For this review, take the finished solid that the model builds, in its own axes (mm). Face numbers are marked on the shaded views. A direction names the side the tool comes from. Coordinates: 2 decimals unless noted, no trailing zeros. Order: outer loops, then holes, each group sorted by start corner. A loop starts at its lowest first (then second) coordinate and runs counter-clockwise, first axis right, second up.
from build123d import *

# Parameters (mm, degrees)
CROQUIS1_R                     = 12.5
CROQUIS1_R_2                   = 11
SALIENTE_EXTRUIR1_DEPTH        = 4
SALIENTE_EXTRUIR1_DEPTH_BACK   = 4
CROQUIS1_R_3                   = 6.5
CROQUIS1_R_4                   = 5
SALIENTE_EXTRUIR1_2_DEPTH      = 4
SALIENTE_EXTRUIR1_2_DEPTH_BACK = 4
CROQUIS1_4_R                   = 11
CROQUIS1_4_R_2                 = 6.5
SALIENTE_EXTRUIR2_DEPTH        = 3.5
SALIENTE_EXTRUIR2_DEPTH_BACK   = 3.5


with BuildPart() as part:
    # Croquis1 → Saliente-Extruir1 (new body, two sides)
    with BuildSketch(Plane.XY) as saliente_extruir1_sk:
        Circle(CROQUIS1_R)
        Circle(CROQUIS1_R_2, mode=Mode.SUBTRACT)
    extrude(amount=SALIENTE_EXTRUIR1_DEPTH)
    extrude(saliente_extruir1_sk.sketch, amount=-SALIENTE_EXTRUIR1_DEPTH_BACK)



with BuildPart() as body_2:
    # Croquis1 → Saliente-Extruir1 2 (new body, two sides)
    with BuildSketch(Plane.XY) as saliente_extruir1_2_sk:
        Circle(CROQUIS1_R_3)
        Circle(CROQUIS1_R_4, mode=Mode.SUBTRACT)
    extrude(amount=SALIENTE_EXTRUIR1_2_DEPTH)
    extrude(saliente_extruir1_2_sk.sketch, amount=-SALIENTE_EXTRUIR1_2_DEPTH_BACK)


with BuildPart() as part_1:
    add(part.part)

    add(body_2.part)  # Saliente-Extruir2 merges body 2
    # Croquis1_4 → Saliente-Extruir2 (add, two sides)
    with BuildSketch(Plane.XY) as saliente_extruir2_sk:
        Circle(CROQUIS1_4_R)
        Circle(CROQUIS1_4_R_2, mode=Mode.SUBTRACT)
    extrude(amount=SALIENTE_EXTRUIR2_DEPTH)
    extrude(saliente_extruir2_sk.sketch, amount=-SALIENTE_EXTRUIR2_DEPTH_BACK)


solid = part_1.part
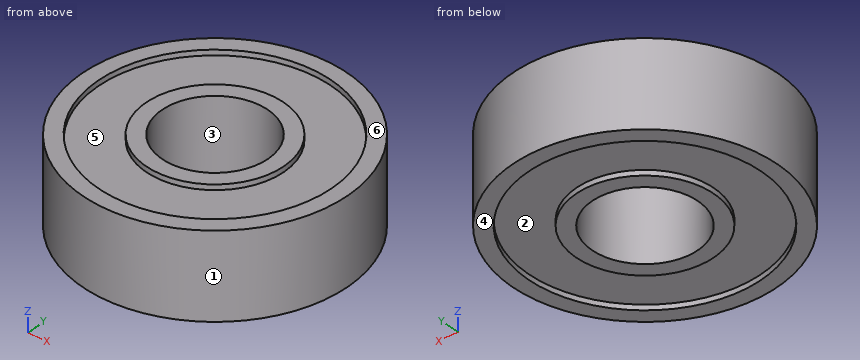
1. Clearance check with flat-ended pins moving along their axes: pin 1 Ø1.5 at (x, y) = (-9, -5.5) entering from +Z; pin 2 Ø2 at (x, y) = (-8, 5.5) entering from -Z; pin 3 Ø6 at (x, y) = (0, 0) entering from -Z. State where each tip first meets the part, or that it passes through.
Answer below:
pin 1: stops at z = 4
pin 2: stops at z = -3.5
pin 3: passes through
2. Take a section at D-D, the plane z = 0.25. Give the boundary of the cut face in (x, y).
Answer below:
outline: circle Ø25 at (0, 0); hole circle Ø10 at (0, 0)
3. Machinability: for the marked faces 5 and 6, which of the approach directions +Z, -Z, +X, -X, +Y, -Y give a long, thin tool a straight path to every point of the face, cutting with its end or side? Answer none if there is none.
Answer below:
face 5: +Z
face 6: +Z, +X, -X, +Y, -Y
4. The part is to be moulded in two halves that separate along X. For the marked faces 1, 2, 3 and 4, say which applies: +X half, -X half, draft (parallel to the pull), parting line (faces both ways), or undercut.
Answer below:
face 1: parting line
face 2: undercut
face 3: undercut
face 4: draft
5. Take a section at C-C, the plane y = -7.5. Give the boundary of the cut face in (x, z), plus the area to 3 significant figures.
Answer below:
outline: (-10, -4) - (-8.05, -4) - (-8.05, -3.5) - (8.05, -3.5) - (8.05, -4) - (10, -4) - (10, 4) - (8.05, 4) - (8.05, 3.5) - (-8.05, 3.5) - (-8.05, 4) - (-10, 4) - close
area: 144 mm2
6. Take a section at A-A, the plane x = 0. Give the boundary of the cut face in (y, z).
Answer below:
outline: (-12.5, -4) - (-11, -4) - (-11, -3.5) - (-6.5, -3.5) - (-6.5, -4) - (-5, -4) - (-5, 4) - (-6.5, 4) - (-6.5, 3.5) - (-11, 3.5) - (-11, 4) - (-12.5, 4) - close; (5, -4) - (6.5, -4) - (6.5, -3.5) - (11, -3.5) - (11, -4) - (12.5, -4) - (12.5, 4) - (11, 4) - (11, 3.5) - (6.5, 3.5) - (6.5, 4) - (5, 4) - close
7. To check wall thickness, follow L1, parallel to Y at x = 0, z = -3.55; L2, parallel to Y at x = 0, z = -1; L3, parallel to Z at x = -2.5, y = -7.25. State the ranges of each line that lie inside material, in increasing order.
Answer below:
L1: y = -12.5 to -11, -6.5 to -5, 5 to 6.5, 11 to 12.5
L2: y = -12.5 to -5, 5 to 12.5
L3: z = -3.5 to 3.5
